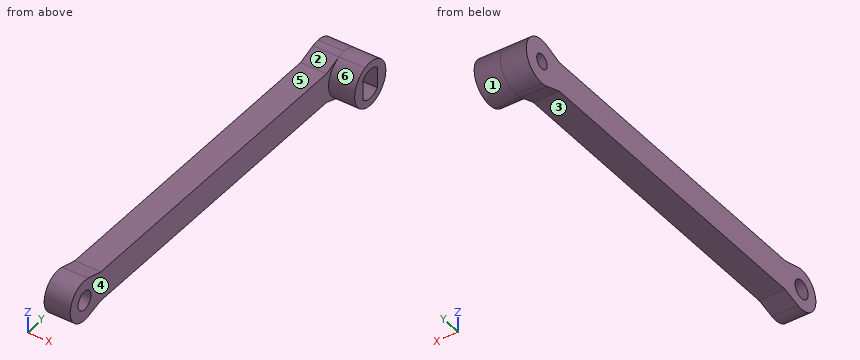
Autodesk Inventor part; units mm, degrees
ref_plane "YZ Plane" through (0, 0, 0) normal (1, 0, 0) x (0, 1, 0)
ref_plane "XZ Plane" through (0, 0, 0) normal (0, 1, 0) x (-1, 0, 0)
ref_plane "XY Plane" through (0, 0, 0) normal (0, 0, 1) x (1, 0, 0)
sketch "Sketch1" plane through (0, 0, 0) normal (1, 0, 0) x (0, 1, 0)
  line L0 (-39.2, 0) -> (39.2, 0)
  line L1 (0, -4.2) -> (0, 4.2)
  circle A0 centre (-25, 0) radius 1.25
  circle A1 centre (-25, 0) radius 3
  circle A2 centre (25, 0) radius 3 construction
  line L2 (-25, 3) -> (25, 3)
  line L3 (-25, -3) -> (25, -3)
  line L4 (25, 3) -> (25, -3) construction
  line L5 (25, 2) -> (25, -2) construction
  arc A3 (25, -3) -> (25, 3) centre (25, 0) ccw
  circle A4 centre (-25, 0) radius 2.2678 construction
  circle A5 centre (25, 0) radius 1
  point P0 (0, 0)
  point P1 (25, 0)
  dimension "d4" = 6
  dimension "d7" = 50
  dimension "d8" = 2.5
  dimension "d10" = 0
  dimension "d30" = 2
extrude "ext_main" add sketch "Sketch1" along normal mid plane 3.5 contours A0 L0 A1 | L0 A1 A0 | A1 L2 L1 L0 | L0 L1 L3 A1 | L1 L2 A3 L0 A5 | L0 A5 A3 L3 L1
sketch "Sketch3" plane through (0, 0, 0) normal (1, 0, 0) x (0, 1, 0)
  arc A0 (-25, 3) -> (-25, -3) centre (-25, 0) ccw
  circle A1 centre (-25, 0) radius 1.25
  arc A2 (25, -3) -> (25, 3) centre (25, 0) ccw
  circle A3 centre (-25, 0) radius 3 construction
  circle A4 centre (25, 0) radius 3 construction
  line L0 (-22.7639, 2) -> (22.7639, 2) construction
  line L1 (-39.2, 0) -> (39.2, 0)
  line L2 (0, -4.2579) -> (0, 4.2579)
  line L3 (25, 3) -> (-25, 3)
  line L4 (21.6192, 2) -> (24.0141, 2.8334)
  arc A5 (25, 3) -> (24.0141, 2.8334) centre (25, 0) ccw
  line L5 (-21.8389, 2) -> (21.6192, 2)
  circle A6 centre (-25, 0) radius 2.75
  line L6 (-21.8389, 2) -> (-24.2882, 2.6563)
  arc A7 (24.0141, -2.8334) -> (25, -3) centre (25, 0) ccw
  line L7 (21.6192, -2) -> (-22.7639, -2) construction
  line L8 (-21.8389, -2) -> (-24.2882, -2.6563)
  line L9 (21.6192, -2) -> (-21.8389, -2)
  line L10 (21.6192, -2) -> (24.0141, -2.8334)
  point P0 (0, 0)
  dimension "d16" = 1
  dimension "d21" = 5.5
  dimension "d22" = 15
extrude "ext_cutaway" cut sketch "Sketch3" along normal through all both and the other way through all contours A6 L1 A1 | L1 A1 A6 | L5 L4 A5 A2 L1 L2 | L2 L1 A6 L6 L5 | A6 L1 L2 L9 L8 | L1 A2 A7 L10 L9 L2 keep common part
sketch "Sketch4" plane through (1.75, 0, 0) normal (1, 0, 0) x (0, 0, -1)
  arc A0 (2.8334, 24.0141) -> (-2.8334, 24.0141) centre (0, 25) ccw
  circle A1 centre (0, 25) radius 1
  circle A2 centre (0, 25) radius 3
  line L0 (-4.2, 0) -> (4.2, 0)
  line L1 (-3, 25) -> (3, 25) construction
  circle A3 centre (0, 25) radius 2 construction
  arc A4 (-1.4283, 26.4) -> (-1.4283, 23.6) centre (0, 25) ccw
  arc A5 (1.4283, 23.6) -> (1.4283, 26.4) centre (0, 25) ccw
  line L2 (-1.4283, 26.4) -> (1.4283, 26.4)
  line L3 (-1.4283, 23.6) -> (1.4283, 23.6)
  point P0 (0, 0)
  dimension "d23" = 4
  dimension "d25" = 2.8
extrude "ext_potshaft" add sketch "Sketch4" along normal blind 3.5 contours A2 A0
extrude "ext_cut_potshaft" cut sketch "Sketch4" against normal blind 1 contours L2 A5 L3 A4
equation "\"d7\" = general_link_length"
equation "\"d8\" = screw_m2_bore_loose"
equation "\"d30\" = screw_m2_bore_selfthreading"
equation "\"d21\" = general_bore_smallersupport_diameter"
properties part number "empty"
Build history of the part. All positions in model axes, mm. Face numbers are marked on the shaded views. A direction names the side the tool comes from. Give positions to 0.01 mm unless a question says otherwise; leave off trailing zeros. Loops run counter-clockwise (first coordinate to the right, second up) from the corner with the lowest first, then second, coordinate; pieces in that order, holes last. Notation, with made-up numbers: (81, 5.5) -> (129, 5.5) arc R17 cw to (129, 14.5) -> close; hole circle Ø3 at (51.25, 13.25). An arc over 180 degrees is marked (long way). One line per question, with ' | ' between items. Start each with the question number.
1) 3-axis set-ups, long thin cutter, end or side, ignore diameter. For the marked faces 1, 2 and 3: which of +Z, -Z, +X, -X, +Y, -Y reach the whole face in a straight line?
2) Cut at B-B (z = 0). Give the cut face in (x, y).
3) Pin check, flat tips, straight feed: pin 1 (1 mm diameter, centred on x = 1.5, y = 19.5, fed in from +Z); pin 2 (1.8 mm diameter, centred on x = 1, y = 8, fed in from -Z); pin 3 (3 mm diameter, centred on y = -14, z = -1.5, fed in from +X). Stop position of each tip, or through.
4) Cut at A-A (x = 4.5). Give the cut face in (y, z).
5) Cut at C-C (x = -0.75). Give the cut face in (y, z), plus the area to 3 significant figures.
6) Two-plate mould, pull along Y, no slides. Class the marked faces 4, 5 and 6: released by +Y, released by -Y, zero draft, split by the parting line, or undercut.
7) Probe L1, parallel to Y at x = 0.9, z = 0; L2, parallel to Z at x = -0.25, y = -25; L3, parallel to Z at x = -0.5, y = 16. List the from-to ranges inside material, lowest first.
8) Cut at D-D (y = -3). Give the cut face in (x, z), plus the area to 3 significant figures.
Return value:
1) face 1: +X, -X | face 2: +Z, +X, -X | face 3: -Z, +X, -X
2) outline: (-1.75, -27.75) -> (1.75, -27.75) -> (1.75, -26.25) -> (-1.75, -26.25) -> close; (-1.75, -23.75) -> (1.75, -23.75) -> (1.75, 22) -> (5.25, 22) -> (5.25, 23.6) -> (0.75, 23.6) -> (0.75, 24) -> (-1.75, 24) -> close; (-1.75, 26) -> (0.75, 26) -> (0.75, 26.4) -> (5.25, 26.4) -> (5.25, 28) -> (-1.75, 28) -> close
3) pin 1: z = 2 | pin 2: z = -2 | pin 3: x = 1.75
4) outline: circle Ø6 at (25, 0); hole (23.6, -1.43) arc R2 ccw to (26.4, -1.43) -> (26.4, 1.43) arc R2 ccw to (23.6, 1.43) -> close
5) outline: (-24.29, -2.66) -> (-21.84, -2) -> (21.62, -2) -> (24.01, -2.83) arc R3 ccw to (25, -3) arc R3 ccw to (25, 3) arc R3 ccw to (24.01, 2.83) -> (21.62, 2) -> (-21.84, 2) -> (-24.29, 2.66) arc R2.75 ccw (long way) to start; hole circle Ø2.5 at (-25, 0); hole circle Ø2 at (25, 0) | area: 224 mm^2
6) face 4: zero draft | face 5: undercut | face 6: released by -Y
7) L1: -27.75 to -26.25, -23.75 to 23.6, 26.4 to 28 | L2: -2.75 to -1.25, 1.25 to 2.75 | L3: -2 to 2
8) outline: (-1.75, -2) -> (1.75, -2) -> (1.75, 2) -> (-1.75, 2) -> close | area: 14.0 mm^2
